```python
from build123d import *

# Parameters (mm, degrees)
SKETCH_1_W          = 7
SKETCH_1_H          = 24
SKETCH_1_R          = 1.55
EXTRUDE_1_DEPTH     = 9
SKETCH_2_W          = 7
SKETCH_2_H          = 12
EXTRUDE_2_DEPTH     = 11
SKETCH_3_R          = 1.55
CUT_EXTRUDE_1_DEPTH = 5


with BuildPart() as part:
    # 草图1 → 凸台-拉伸1 (new body)
    with BuildSketch(Plane.XY):
        with Locations((3.525062814, 16.5)):
            Rectangle(SKETCH_1_W, SKETCH_1_H)
        with Locations((3, 24.5)):
            Circle(SKETCH_1_R, mode=Mode.SUBTRACT)
    extrude(amount=EXTRUDE_1_DEPTH)

    # 草图2 → 凸台-拉伸2 (add)
    with BuildSketch(Plane.XY.offset(9)):
        with Locations((3.525062814, 10.5)):
            Rectangle(SKETCH_2_W, SKETCH_2_H)
    extrude(amount=EXTRUDE_2_DEPTH)

    # 草图3 → 切除-拉伸1 (cut)
    with BuildSketch(Plane(origin=(0, 4.5, 0), x_dir=(-1, 0, 0), z_dir=(0, -1, 0))):
        with Locations(Location((-3.525062814, -5, 0), (0, 0, 180))):
            Circle(SKETCH_3_R)
        with Locations(Location((-3.525062814, -15, 0), (0, 0, 180))):
            Circle(SKETCH_3_R)
    extrude(amount=-CUT_EXTRUDE_1_DEPTH, mode=Mode.SUBTRACT)


solid = part.part
```
Work out the finished part from the listing and answer in its coordinate system (mm). A direction names the side the tool comes from. Coordinates: 2 decimals unless noted, no trailing zeros. Loops run counter-clockwise (first coordinate to the right, second up) from the corner with the lowest first, then second, coordinate; pieces in that order, holes last. Notation, with made-up numbers: (-22, 8.25) - (3, 8.25) arc R10 cw to (3, 12.25) - close; hole circle Ø3 at (19.25, -17.75). An arc over 180 degrees is marked (long way). Use a Markdown table: item, result.
Item 1: Find section A-A, the plane x = 3. Determine the outline of the cut face in (y, z), and give its area (3 significant figures).
Evaluation:
| item | result |
|---|---|
| outline | (4.5, 0) - (22.95, 0) - (22.95, 9) - (16.5, 9) - (16.5, 20) - (4.5, 20) - (4.5, 16.46) - (9.5, 16.46) - (9.5, 13.54) - (4.5, 13.54) - (4.5, 6.46) - (9.5, 6.46) - (9.5, 3.54) - (4.5, 3.54) - close; (26.05, 0) - (28.5, 0) - (28.5, 9) - (26.05, 9) - close |
| area | 291 mm2 |
Item 2: Find section C-C, the plane y = 8.25. Determine the outline of the cut face in (x, z).
Evaluation:
| item | result |
|---|---|
| outline | (0.03, 0) - (7.03, 0) - (7.03, 20) - (0.03, 20) - close; hole circle Ø3.1 at (3.53, 5); hole circle Ø3.1 at (3.53, 15) |
Item 3: Given pin 1 Ø2 at (x, y) = (3, 23.5) entering from +Z; pin 2 Ø2 at (x, z) = (5.5, 16) entering from +Y, each flat-ended and moving along its own axis, determine where each tip first touches the part or whether it passes through.
Evaluation:
| item | result |
|---|---|
| pin 1 | stops at z = 9 |
| pin 2 | stops at y = 16.5 |
Item 4: For faces 1 (the flat face through (3, 16.5, 14)), 2 (the flat face through (3, 4.5, 10)), 3 (the flat face through (4, 9.5, 5)), determine the directions among +Z, -Z, +X, -X, +Y, -Y from which every point of the face is accessible in a straight line to the end or side of a thin tool.
Evaluation:
| item | result |
|---|---|
| face 1 | +Z, +X, -X, +Y |
| face 2 | +Z, -Z, +X, -X, -Y |
| face 3 | -Y |
Item 5: The mould has two halves that part along X. Classify faces 4 (the cylindrical face through (2.798, 26.037, 4.437)), 5 (the flat face through (7.025, 14, 8)), 6 (the flat face through (3, 17, 0)): +X half, -X half, draft (parallel to the pull), parting line (faces both ways), or undercut.
Evaluation:
| item | result |
|---|---|
| face 4 | undercut |
| face 5 | +X half |
| face 6 | draft |
Item 6: Find section B-B, the plane z = 5. Determine the outline of the cut face in (x, y).
Evaluation:
| item | result |
|---|---|
| outline | (0.03, 4.5) - (1.98, 4.5) - (1.98, 9.5) - (5.08, 9.5) - (5.08, 4.5) - (7.03, 4.5) - (7.03, 28.5) - (0.03, 28.5) - close; hole circle Ø3.1 at (3, 24.5) |
Item 7: Find section D-D, the plane z = 15. Determine the outline of the cut face in (x, y), and give its area (3 significant figures).
Evaluation:
| item | result |
|---|---|
| outline | (0.03, 4.5) - (1.98, 4.5) - (1.98, 9.5) - (5.08, 9.5) - (5.08, 4.5) - (7.03, 4.5) - (7.03, 16.5) - (0.03, 16.5) - close |
| area | 68.5 mm2 |
Item 8: Consider probe 1 along Y at (x, z) = (3, 4); probe 2 along Z at (x, y) = (2, 17.25); probe 3 along Y at (x, z) = (4, 10). Determine where each line is inside the solid, lowest interval first. Write a range as from..to.
Evaluation:
| item | result |
|---|---|
| probe 1 | y = 9.5..22.95, 26.05..28.5 |
| probe 2 | z = 0..9 |
| probe 3 | y = 4.5..16.5 |
